from build123d import *

# Parameters (mm, degrees)
F0_R     = 14.9287421436
F1_DEPTH = 38.1
F0_W     = 91.0995900631
F0_H     = 68.1872144341
F2_DEPTH = 25.4
F3_DEPTH = 12.7
F5_DEPTH = 25.4


with BuildPart() as f1:
    # F0 (on Top) → F1 (new body)
    with BuildSketch(Plane.XY):
        Circle(F0_R)
    extrude(amount=F1_DEPTH)

    # F0 (on Top) → F2 (join)
    with BuildSketch(Plane.XY):
        Rectangle(F0_W, F0_H)
        Circle(F0_R, mode=Mode.SUBTRACT)
    extrude(amount=F2_DEPTH)

    # F3 (add): a face of the model
    f3_faces = [f1.faces().sort_by_distance(p)[0] for p in [
        (0, 0, 38.1),
    ]]
    extrude(f3_faces, amount=F3_DEPTH)

    # F4 (on Right) → F5 (cut, symmetric)
    with BuildSketch(Plane.YZ):
        Polygon((-16.5885575116, 54.623093456), (-16.4052583277, 50.4072159529), (20.9877323359, 32.0773199201), (20.9877323359, 54.623093456), align=None)
    extrude(amount=F5_DEPTH, both=True, mode=Mode.SUBTRACT)


solid = f1.part
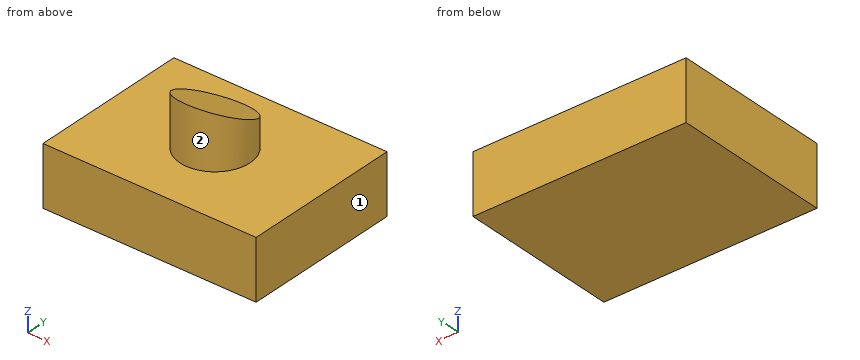
The listing builds one solid part. Answer for the finished solid, in the listing's coordinates (mm). Face numbers are marked on the shaded views. A direction names the side the tool comes from. Round coordinates to 2 decimals unless told otherwise and drop trailing zeros. Order: outer loops, then holes, each group sorted by start corner. A loop starts at its lowest first (then second) coordinate and runs counter-clockwise, first axis right, second up. Notation, with made-up numbers: (38, 35) -> (97, 35) arc R22 ccw to (97, 57) -> close; hole circle Ø3 at (-23, 64). An arc over 180 degrees is marked (long way). Write each question's results on one line, items separated by ' | '. Start each with the question number.
Q1. Straight lines are drawn through the part: probe 1 along Z at (x, y) = (20.5, -15); probe 2 along Y at (x, z) = (-11, 45); probe 3 along X at (y, z) = (-10, 29.5). For each, find the intervals that lie inside material, in ascending order. Write a range as from..to.
Q2. Find section C-C (z = 30). Determine the outline of the cut face in (x, y).
Q3. Find section B-B (y = 0). Determine the outline of the cut face in (x, z).
Q4. This flat-tipped pin is pushed along its axis until it touches: pin 1 (6 mm diameter, centred on x = -19, y = -23, fed in from +Z). Where does it stop, or does it pass through?
Q5. Which of the six approach directions +Z, -Z, +X, -X, +Y, -Y give full straight-line access (tool end or side, diameter ignored) to the marked faces 1 and 2?
Q6. Find section A-A (x = 0). Determine the outline of the cut face in (y, z).
Q7. Find section D-D (y = 26). Determine the outline of the cut face in (x, z).
Worked answers:
1) probe 1: z = 0..25.4 | probe 2: y = -10.09..-5.37 | probe 3: x = -11.08..11.08
2) outline: circle Ø29.86 at (0, 0)
3) outline: (-45.55, 0) -> (45.55, 0) -> (45.55, 25.4) -> (14.93, 25.4) -> (14.93, 42.37) -> (-14.93, 42.37) -> (-14.93, 25.4) -> (-45.55, 25.4) -> close
4) pin 1: stops at z = 25.4
5) face 1: +Z, -Z, +X, +Y, -Y | face 2: +Z
6) outline: (-34.09, 0) -> (34.09, 0) -> (34.09, 25.4) -> (14.93, 25.4) -> (14.93, 35.05) -> (-14.93, 49.68) -> (-14.93, 25.4) -> (-34.09, 25.4) -> close
7) outline: (-45.55, 0) -> (45.55, 0) -> (45.55, 25.4) -> (-45.55, 25.4) -> close
